Part print with two shaded views. Sizes in mm from the minimum x, y, z corner. A direction names the side the tool comes from. Round coordinates to 2 decimals unless told otherwise and drop trailing zeros. Order: outer loops, then holes, each group sorted by start corner. A loop starts at its lowest first (then second) coordinate and runs counter-clockwise, first axis right, second up. Notation, with made-up numbers: (18.25, -18.75) -> (63.25, -18.75) arc R30 ccw to (63.25, 18.25) -> close; hole circle Ø3 at (84.25, 5). An arc over 180 degrees is marked (long way). Use a Markdown table: item, result. Add a question column.
Item 1: Slice it at C-C, the plane z = 6. Give the cut face in (x, y).
Item 2: Two-plate mould, pull along X, no slides. Class the marked faces 3, 4, 5 and 6: released by +X, released by -X, zero draft, split by the parting line, or undercut.
Item 3: Probe L1, parallel to X at y = 7.5, z = 44; L2, parallel to X at y = 7.75, z = 7; L3, parallel to Y at x = 69, z = 11.55. List the from-to ranges inside material, lowest first.
Item 4: 3-axis set-ups, long thin cutter, end or side, ignore diameter. For the marked faces 1 and 2: which of +Z, -Z, +X, -X, +Y, -Y reach the whole face in a straight line?
Item 5: Pin check, flat tips, straight feed: pin 1 (5 mm diameter, centred on y = 5, z = 6.5, fed in from +X); pin 2 (5 mm diameter, centred on y = 2.5, z = 6, fed in from -X); pin 3 (3 mm diameter, centred on x = 69, y = 5, fed in from -Z). Stop position of each tip, or through.
Item 6: Slice it at D-D, the plane y = 9. Give the cut face in (x, z), plus the area to 3 significant figures.
Item 7: Slice it at A-A, the plane x = 6. Give the cut face in (y, z).
Item 8: Slice it at B-B, the plane z = 44. Give the cut face in (x, y), plus the area to 3 significant figures.
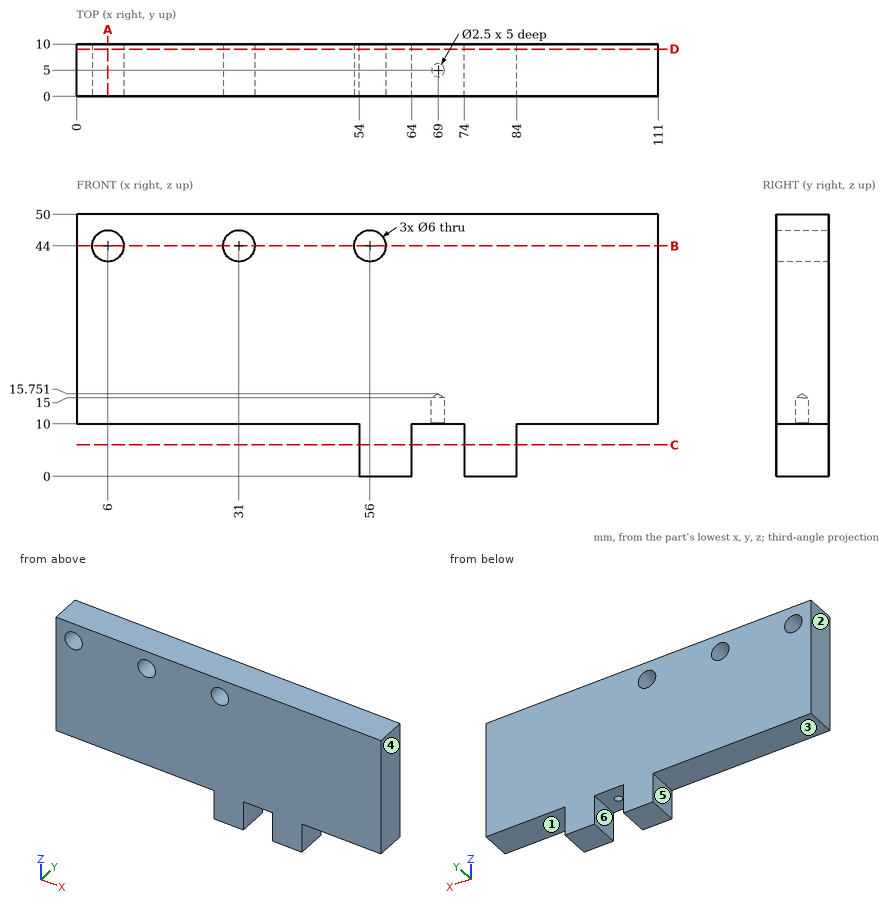
Check sheet entries:
| question | item | result |
|---|---|---|
| 1 | outline | (54, 0) -> (64, 0) -> (64, 10) -> (54, 10) -> close; (74, 0) -> (84, 0) -> (84, 10) -> (74, 10) -> close |
| 2 | face 3 | zero draft |
| 2 | face 4 | released by +X |
| 2 | face 5 | released by -X |
| 2 | face 6 | undercut |
| 3 | L1 | 0 to 3, 9 to 28, 34 to 53, 59 to 111 |
| 3 | L2 | 54 to 64, 74 to 84 |
| 3 | L3 | 0 to 3.75, 6.25 to 10 |
| 4 | face 1 | -Z, +X, +Y, -Y |
| 4 | face 2 | +Z, -Z, -X, +Y, -Y |
| 5 | pin 1 | x = 84 |
| 5 | pin 2 | x = 54 |
| 5 | pin 3 | z = 10 |
| 6 | outline | (0, 10) -> (54, 10) -> (54, 0) -> (64, 0) -> (64, 10) -> (74, 10) -> (74, 0) -> (84, 0) -> (84, 10) -> (111, 10) -> (111, 50) -> (0, 50) -> close; hole circle Ø6 at (6, 44); hole circle Ø6 at (31, 44); hole circle Ø6 at (56, 44) |
| 6 | area | 4,560 mm2 |
| 7 | outline | (0, 10) -> (10, 10) -> (10, 41) -> (0, 41) -> close; (0, 47) -> (10, 47) -> (10, 50) -> (0, 50) -> close |
| 8 | outline | (0, 0) -> (3, 0) -> (3, 10) -> (0, 10) -> close; (9, 0) -> (28, 0) -> (28, 10) -> (9, 10) -> close; (34, 0) -> (53, 0) -> (53, 10) -> (34, 10) -> close; (59, 0) -> (111, 0) -> (111, 10) -> (59, 10) -> close |
| 8 | area | 930 mm2 |
